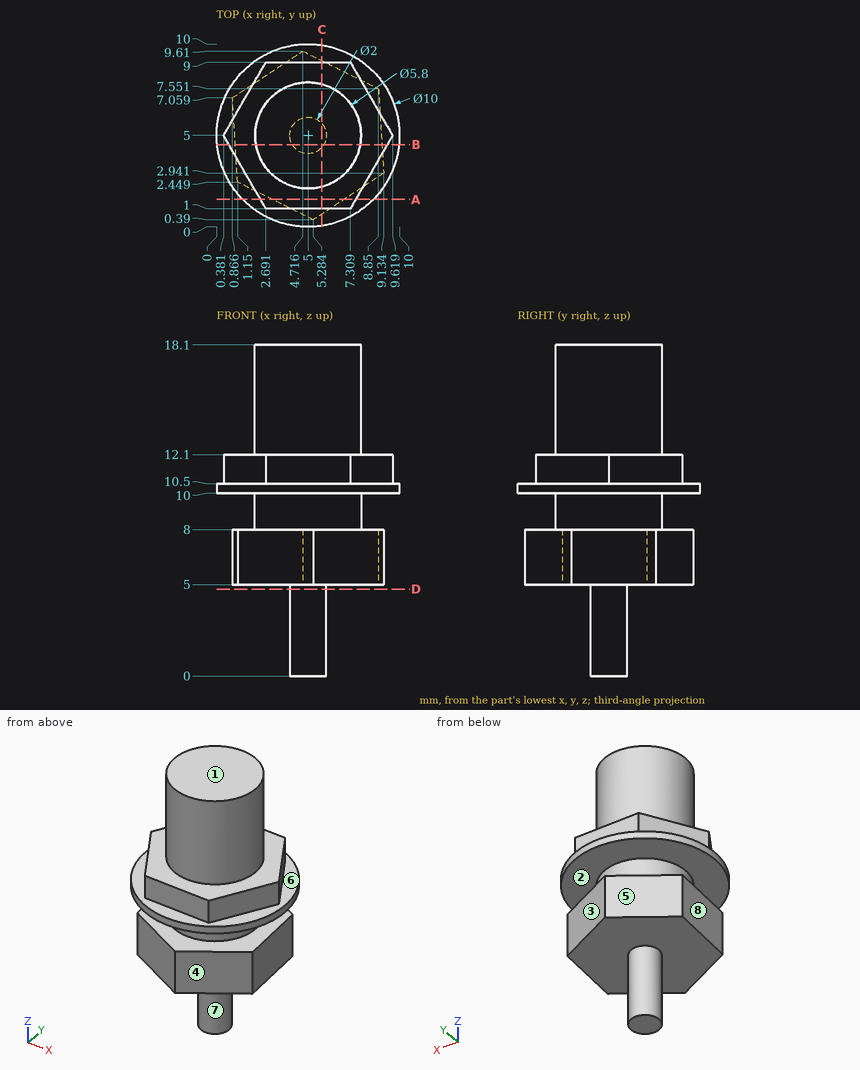
Job drawing, mm, ordinate dimensions from the low corner. One solid piece. A direction names the side the tool comes from. Give positions to 0.01 mm unless a question says otherwise; leave off trailing zeros. Order: outer loops, then holes, each group sorted by start corner. A loop starts at its lowest first (then second) coordinate and runs counter-clockwise, first axis right, second up. Notation, with made-up numbers: (-36, 78.5) - (-1, 78.5) arc R18 ccw to (-1, 108.5) - close; hole circle Ø9 at (16, 43). An arc over 180 degrees is marked (long way). Answer in a Markdown table with one row per item.
1. Saw through at B-B, the plane y = 4.5. Give the cut face in (x, z) (1 decimal).
Data:
| item | result |
|---|---|
| outline | (0, 10) - (2.1, 10) - (2.1, 8) - (1, 8) - (1, 5) - (4.1, 5) - (4.1, 0) - (5.9, 0) - (5.9, 5) - (9, 5) - (9, 8) - (7.9, 8) - (7.9, 10) - (10, 10) - (10, 10.5) - (9.3, 10.5) - (9.3, 12.1) - (7.9, 12.1) - (7.9, 18.1) - (2.1, 18.1) - (2.1, 12.1) - (0.7, 12.1) - (0.7, 10.5) - (0, 10.5) - close |
2. Saw through at D-D, the plane z = 4.75. Give the cut face in (x, y).
Data:
| item | result |
|---|---|
| outline | circle Ø2 at (5, 5) |
3. Probe probe 1 along Z at (x, y) = (6.5, 1.75); probe 2 along Z at (x, y) = (6.5, 0.5); probe 3 along Y at (x, z) = (6.5, 10.75). List the from-to ranges inside material, lowest first. Write a range as [from, to].
Data:
| item | result |
|---|---|
| probe 1 | z = [5, 8], [10, 12.1] |
| probe 2 | z = [10, 10.5] |
| probe 3 | y = [1, 9] |
4. Pull direction Z, two halves, no side cores. Call the marked faces 1, 2 and 3: pulls with the +Z half, pulls with the -Z half, needs draft (parallel to the pull), parting line crosses it, or undercut.
Data:
| item | result |
|---|---|
| face 1 | pulls with the +Z half |
| face 2 | undercut |
| face 3 | needs draft |
5. Flat gauge pins, fed straight in: pin 1 (5 mm diameter, centred on y = 7, z = 2, fed in from -X); pin 2 (1.3 mm diameter, centred on x = 5.5, z = 11, fed in from +Y); pin 3 (2 mm diameter, centred on x = 2, y = 1.5, fed in from +Z); pin 4 (1.5 mm diameter, centred on y = 5, z = 9, fed in from -X). Where does each tip first touch, or does it go through?
Data:
| item | result |
|---|---|
| pin 1 | stops at x = 4 |
| pin 2 | stops at y = 10 |
| pin 3 | stops at z = 12.1 |
| pin 4 | stops at x = 2.1 |
6. Tool access for the marked faces 4, 5, 6, 7 and 8: list every direction of +Z, -Z, +X, -X, +Y, -Y with a clear straight run to the whole face (end or side of a thin tool).
Data:
| item | result |
|---|---|
| face 4 | -Z, +X, -Y |
| face 5 | -Z, -X, +Y |
| face 6 | +Z |
| face 7 | -Z |
| face 8 | -Z, -X, -Y |
7. Saw through at A-A, the plane y = 1.5. Give the cut face in (x, z) (1 decimal).
Data:
| item | result |
|---|---|
| outline | (1.4, 10) - (8.6, 10) - (8.6, 10.5) - (7.6, 10.5) - (7.6, 12.1) - (2.4, 12.1) - (2.4, 10.5) - (1.4, 10.5) - close; (3.1, 5) - (7, 5) - (7, 8) - (3.1, 8) - close |
8. Saw through at C-C, the plane x = 5.75. Give the cut face in (y, z) (1 decimal).
Data:
| item | result |
|---|---|
| outline | (0.1, 10) - (2.2, 10) - (2.2, 8) - (0.7, 8) - (0.7, 5) - (4.3, 5) - (4.3, 0) - (5.7, 0) - (5.7, 5) - (9.1, 5) - (9.1, 8) - (7.8, 8) - (7.8, 10) - (9.9, 10) - (9.9, 10.5) - (9, 10.5) - (9, 12.1) - (7.8, 12.1) - (7.8, 18.1) - (2.2, 18.1) - (2.2, 12.1) - (1, 12.1) - (1, 10.5) - (0.1, 10.5) - close |
